```python
from build123d import *

# Parameters (mm, degrees)
SKETCH1_R                               = 38.1
BOSS_EXTRUDE1_DEPTH                     = 17.272
CBORE_FOR_M6_HEX_HEAD_BOLT1_D           = 6.6
CBORE_FOR_M6_HEX_HEAD_BOLT1_CBORE_D     = 14.55
CBORE_FOR_M6_HEX_HEAD_BOLT1_CBORE_DEPTH = 4.38
SKETCH6_R                               = 1.515
PIN_FOR_M6_DEPTH                        = 17.272
M5X0_8_TAPPED_HOLE1_D                   = 4.2
SKETCH10_R                              = 1.05
SPRING_PIN_HOLE_DEPTH                   = 17.272
ALLIGNMENT_BORDER_DEPTH                 = 3
CUT_EXTRUDE2_DEPTH                      = 0.9
SKETCH16_R                              = 2.286
R_PIN_GROUNDING_DEPTH                   = 4.318
CUT_EXTRUDE3_START                      = -12.446
CUT_EXTRUDE3_DEPTH                      = 12.446
SKETCH18_W                              = 4.238089583
SKETCH18_H                              = 12.155953692
CUT_EXTRUDE4_DEPTH                      = 5.08
BOSS_EXTRUDE2_START                     = -17.272
SKETCH19_R                              = 1.515
BOSS_EXTRUDE2_DEPTH                     = 17.272
SKETCH20_R                              = 1.524
CUT_EXTRUDE5_DEPTH                      = 5.08


with BuildPart() as part:
    # Sketch1 → Boss-Extrude1 (new body)
    with BuildSketch(Plane.XY):
        Circle(SKETCH1_R)
    extrude(amount=BOSS_EXTRUDE1_DEPTH)

    # CBORE for M6 Hex Head Bolt1 (through all)
    with Locations(Plane.XY.offset(17.272)):
        with Locations((17.67766953, 17.67766953), (17.67766953, -17.67766953), (-17.67766953, -17.67766953), (-17.67766953, 17.67766953)):
            CounterBoreHole(CBORE_FOR_M6_HEX_HEAD_BOLT1_D / 2, CBORE_FOR_M6_HEX_HEAD_BOLT1_CBORE_D / 2, CBORE_FOR_M6_HEX_HEAD_BOLT1_CBORE_DEPTH)

    # Sketch6 → Pin_for_M6 (cut)
    with BuildSketch(Plane.XY.offset(17.272)):
        with Locations((-5.653014274, 24.676900213)):
            Circle(SKETCH6_R)
    extrude(amount=-PIN_FOR_M6_DEPTH, mode=Mode.SUBTRACT)

    # M5x0.8 Tapped Hole1 (through all)
    with Locations(Plane.XY.offset(17.272)):
        with Locations((27.279800219, 15.75), (-27.279800219, 15.75), (27.279800219, -15.75), (-27.279800219, -15.75)):
            Hole(M5X0_8_TAPPED_HOLE1_D / 2)

    # Sketch10 → Spring_Pin_Hole (cut)
    with BuildSketch(Plane.XY.offset(17.272)):
        with Locations((-5.653014274, 24.676900213)):
            Circle(SKETCH10_R)
        with BuildLine():
            Line((-18.212, 3.2385), (-7.188, 3.2385))
            ThreePointArc((-7.188, 3.2385), (-6.05662915, 2.76987085), (-5.588, 1.6385))
            Line((-5.588, 1.6385), (-5.588, -1.6385))
            ThreePointArc((-5.588, -1.6385), (-6.05662915, -2.76987085), (-7.188, -3.2385))
            Line((-7.188, -3.2385), (-18.212, -3.2385))
            ThreePointArc((-18.212, -3.2385), (-19.34337085, -2.76987085), (-19.812, -1.6385))
            Line((-19.812, -1.6385), (-19.812, 1.6385))
            ThreePointArc((-19.812, 1.6385), (-19.34337085, 2.76987085), (-18.212, 3.2385))
        make_face()
    extrude(amount=-SPRING_PIN_HOLE_DEPTH, mode=Mode.SUBTRACT)

    # Sketch13 → Allignment_Border (add)
    with BuildSketch(Plane.XY.offset(17.272)):
        with BuildLine():
            Line((-37.612075155, 6.077976846), (-35.036720701, 6.077976846))
            ThreePointArc((-35.036720701, 6.077976846), (0.151738272, 35.559676257), (35.087315055, 5.778747461))
            ThreePointArc((35.087315055, 5.778747461), (5.928416127, -35.06233709), (-35.036720701, -6.077976846))
            Line((-35.036720701, -6.077976846), (-37.612075155, -6.077976846))
            ThreePointArc((-37.612075155, -6.077976846), (0.15158135, -38.099698465), (37.659246703, -5.778506535))
            ThreePointArc((37.659246703, -5.778506535), (5.928288609, 37.635958792), (-37.612075155, 6.077976846))
        make_face()
    extrude(amount=ALLIGNMENT_BORDER_DEPTH)

    # Sketch15 → Cut-Extrude2 (cut)
    with BuildSketch(Plane.XY.offset(17.272)):
        with BuildLine():
            Line((-20.244, 5.2705), (-5.156, 5.2705))
            ThreePointArc((-5.156, 5.2705), (-4.02462915, 4.80187085), (-3.556, 3.6705))
            Line((-3.556, 3.6705), (-3.556, -3.6705))
            ThreePointArc((-3.556, -3.6705), (-4.02462915, -4.80187085), (-5.156, -5.2705))
            Line((-5.156, -5.2705), (-20.244, -5.2705))
            ThreePointArc((-20.244, -5.2705), (-21.37537085, -4.80187085), (-21.844, -3.6705))
            Line((-21.844, -3.6705), (-21.844, 3.6705))
            ThreePointArc((-21.844, 3.6705), (-21.37537085, 4.80187085), (-20.244, 5.2705))
        make_face()
    extrude(amount=-CUT_EXTRUDE2_DEPTH, mode=Mode.SUBTRACT)

    # Sketch16 → R_Pin_Grounding (cut)
    with BuildSketch(Plane.XY.offset(17.272)):
        with Locations((-30.607, 0)):
            Circle(SKETCH16_R)
    extrude(amount=-R_PIN_GROUNDING_DEPTH, mode=Mode.SUBTRACT)

    # Sketch17 → Cut-Extrude3 (cut)
    with BuildSketch(Plane(origin=(0, 0, 0), x_dir=(-1, 0, 0), z_dir=(0, 0, -1)).offset(CUT_EXTRUDE3_START)):
        with BuildLine():
            Line((-11.43, 12.7), (-35.921024484, 12.7))
            ThreePointArc((-35.921024484, 12.7), (-38.1, 0), (-35.921024484, -12.7))
            Line((-35.921024484, -12.7), (-11.43, -12.7))
            Line((-11.43, -12.7), (-11.43, -19.908773642))
            Line((-11.43, -19.908773642), (11.43, -19.908773642))
            Line((11.43, -19.908773642), (11.43, -12.7))
            Line((11.43, -12.7), (23.368, -12.7))
            Line((23.368, -12.7), (23.368, 12.7))
            Line((23.368, 12.7), (11.43, 12.7))
            Line((11.43, 12.7), (11.43, 19.967789095))
            Line((11.43, 19.967789095), (-11.43, 19.967789095))
            Line((-11.43, 19.967789095), (-11.43, 12.7))
        make_face()
        with BuildLine():
            ThreePointArc((7.188, -3.2385), (6.05662915, -2.76987085), (5.588, -1.6385))
            Line((5.588, -1.6385), (5.588, 1.6385))
            ThreePointArc((5.588, 1.6385), (6.05662915, 2.76987085), (7.188, 3.2385))
            Line((7.188, 3.2385), (18.212, 3.2385))
            ThreePointArc((18.212, 3.2385), (19.34337085, 2.76987085), (19.812, 1.6385))
            Line((19.812, 1.6385), (19.812, -1.6385))
            ThreePointArc((19.812, -1.6385), (19.34337085, -2.76987085), (18.212, -3.2385))
            Line((18.212, -3.2385), (7.188, -3.2385))
        make_face(mode=Mode.SUBTRACT)
    extrude(amount=CUT_EXTRUDE3_DEPTH, mode=Mode.SUBTRACT)

    # Sketch18 → Cut-Extrude4 (cut)
    with BuildSketch(Plane.XY.offset(17.272)):
        with Locations((-37.155765493, 0)):
            Rectangle(SKETCH18_W, SKETCH18_H)
    extrude(amount=-CUT_EXTRUDE4_DEPTH, mode=Mode.SUBTRACT)

    # Sketch19 → Boss-Extrude2 (add)
    with BuildSketch(Plane(origin=(0, 0, 0), x_dir=(-1, 0, 0), z_dir=(0, 0, -1)).offset(BOSS_EXTRUDE2_START)):
        with Locations((5.653014274, 24.676900213)):
            Circle(SKETCH19_R)
    extrude(amount=BOSS_EXTRUDE2_DEPTH)

    # Sketch20 → Cut-Extrude5 (cut)
    with BuildSketch(Plane(origin=(0, 0, 12.446), x_dir=(-1, 0, 0), z_dir=(0, 0, -1))):
        with Locations((8.49829012, -11.272773642)):
            Circle(SKETCH20_R)
        with Locations((8.49829012, 11.331789095)):
            Circle(SKETCH20_R)
    extrude(amount=-CUT_EXTRUDE5_DEPTH, mode=Mode.SUBTRACT)


solid = part.part
```
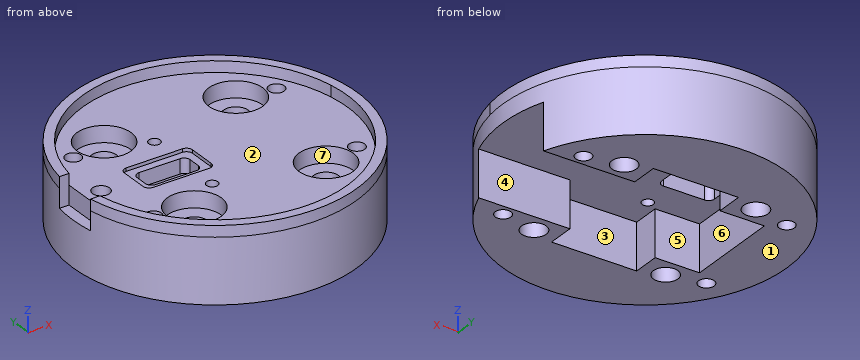
CAD build for the part. Positions are in the model's coordinates, mm. Face numbers are marked on the shaded views. A direction names the side the tool comes from. Round coordinates to 2 decimals unless told otherwise and drop trailing zeros. Order: outer loops, then holes, each group sorted by start corner. A loop starts at its lowest first (then second) coordinate and runs counter-clockwise, first axis right, second up. Notation, with made-up numbers: (54, 5.25) - (83, 5.25) arc R23 ccw to (83, 32.25) - close; hole circle Ø11 at (77.5, -28). An arc over 180 degrees is marked (long way). Use CSV: the item, a comma, the result in double quotes. Start each with the question number.
1) Saw through at C-C (z = 10). Count the separate pieces of the cut face and the enclosed holes in it, and give its area (3 significant figures).
2) Saw through at B-B (x = 0). List the corners of the cut face in (y, z).
3) Tool access for the marked faces 1, 2, 3 and 4: list every direction of +Z, -Z, +X, -X, +Y, -Y with a clear straight run to the whole face (end or side of a thin tool).
4) Saw through at A-A (y = 0). List the corners of the cut face in (x, z).
5) Pin check, flat tips, straight feed: pin 1 Ø1 at (y, z) = (-2.5, 5.5) entering from -X; pin 2 Ø6 at (x, z) = (19, 8) entering from -Y; pin 3 Ø3 at (x, z) = (25, 17) entering from +Y. Stop position of each tip, or through.
6) Two-plate mould, pull along X, no slides. Class the marked faces 5, 6 and 7: pulls with the +X half, pulls with the -X half, needs draft (parallel to the pull), parting line crosses it, or undercut.
7) Wall check: L1, parallel to X at y = -15, z = 15.25; L2, parallel to Y at x = -16, z = 15.5; L3, parallel to Y at x = -19.5, z = 15.5. Give the ranges that are in metal, low to high. Write a range as [from, to].
Values follow:
1,separate pieces,"1"
1,enclosed holes,"8"
1,area,"2,490 mm2"
2,outline,"(-38.1, 0) - (-19.91, 0) - (-19.91, 12.45) - (19.97, 12.45) - (19.97, 0) - (38.1, 0) - (38.1, 20.27) - (35.56, 20.27) - (35.56, 17.27) - (-35.56, 17.27) - (-35.56, 20.27) - (-38.1, 20.27) - close"
3,face 1,"-Z, +X, -X, +Y, -Y"
3,face 2,"+Z"
3,face 3,"-Z"
3,face 4,"-Z, +X"
4,outline,"(-38.1, 0) - (-23.37, 0) - (-23.37, 12.45) - (-19.81, 12.45) - (-19.81, 16.37) - (-21.84, 16.37) - (-21.84, 17.27) - (-28.32, 17.27) - (-28.32, 12.95) - (-32.89, 12.95) - (-32.89, 17.27) - (-35.04, 17.27) - (-35.04, 12.19) - (-38.1, 12.19) - close; (-5.59, 12.45) - (38.1, 12.45) - (38.1, 20.27) - (35.56, 20.27) - (35.56, 17.27) - (-3.56, 17.27) - (-3.56, 16.37) - (-5.59, 16.37) - close"
5,pin 1,"stops at x = -38.05"
5,pin 2,"stops at y = -34.58"
5,pin 3,"stops at y = 29.99"
6,face 5,"needs draft"
6,face 6,"pulls with the +X half"
6,face 7,"undercut"
7,L1,"x = [-35.02, -29.24], [-25.32, -24.44], [-10.91, 10.91], [24.44, 25.32], [29.24, 35.02]"
7,L2,"y = [-34.58, -24.76], [-10.6, -3.24], [3.24, 10.6], [24.76, 34.58]"
7,L3,"y = [-32.73, -24.72], [-10.63, -2.59], [2.59, 10.63], [24.72, 32.73]"
